Input: part model. Units: mm. Frame: model coordinates. Give positions to 0.01 mm unless a question says otherwise; leave off trailing zeros. Loops run counter-clockwise (first coordinate to the right, second up) from the corner with the lowest first, then second, coordinate; pieces in that order, holes last. Notation, with made-up numbers: M 35,53.5 L 92,53.5 A13 ccw 92,62.5 Z; hole C 1,40.25 d3. An arc over 180 degrees is marked long. Answer as a JSON object with one key per item and string values. Group by question number.
1) First-contact query: P1, Ø3, axis at x = 21.5, z = 0.5, coming from the -Y side; P2, Ø2, axis at y = -2, z = -0.5, coming from the +X side; P3, Ø3, axis at y = -1.5, z = 1.5, coming from the -X side; P4, Ø3, axis at x = 0, y = -2, coming from the +Z side. Flat tips, straight axial feed; report the tip coordinate or a pass-through.
2) Section query C-C on x = 24. Return loops of the section in (y, z), plus the area to 3 significant figures.
3) Section query A-A on z = 0. Return loops of the section in (x, y).
4) Draft query along Y for faces 1 (the cylindrical face through (9, 0, 2)), 2 (the flat face through (27.508, 1, 2)), 3 (the cylindrical face through (-9.03, -0.19, 0.03)). Return one class per face: +Y half, -Y half, draft (parallel to the pull), parting line (faces both ways), or undercut.
5) Section query B-B on y = 0. Return loops of the section in (x, z).
6) Ray query, L1, parallel to X at y = 0, z = -0.45; L2, parallel to X at y = 0, z = 1.2; L3, parallel to Y at x = 13, z = 0. Return the intervals inside material, ascending.
from build123d import *

# Parameters (mm, degrees)
SKETCH2_R          = 0.5
CUT_EXTRUDE1_DEPTH = 5
CHAMFER1_SIZE      = 0.5


with BuildPart() as part:
    # Sketch1 → Revolve1 (revolve)
    with BuildSketch(Plane.XY):
        with BuildLine():
            Line((-11.492242367, 0), (-11.492242367, -2))
            Line((-11.492242367, -2), (27.507757633, -2))
            Line((27.507757633, -2), (27.507757633, -3))
            ThreePointArc((27.507757633, -3), (29.629077976, -2.121320344), (30.507757633, 0))
            Line((30.507757633, 0), (-11.492242367, 0))
        make_face()
    revolve(axis=Axis((-20.421686747, 0, 0), (1, 0, 0)))

    # Sketch2 → Cut-Extrude1 (cut, symmetric)
    with BuildSketch(Plane.XY):
        with Locations((-9.492242367, 0)):
            Circle(SKETCH2_R)
    extrude(amount=CUT_EXTRUDE1_DEPTH, both=True, mode=Mode.SUBTRACT)

    # Chamfer1
    chamfer1_edges = [part.edges().sort_by_distance(p)[0] for p in [
        (-11.492242367, 2, 0),
    ]]
    chamfer(chamfer1_edges, length=CHAMFER1_SIZE)


solid = part.part
Output:
{
 "1": {"P1": "stops at y = -2", "P2": "stops at x = 30.31", "P3": "stops at x = -11.49", "P4": "stops at z = 1.94"},
 "2": {"outline": "C 0,0 d4", "area": "12.6 mm^2"},
 "3": {"outline": "M -11.49,-1.5 L -10.99,-2 L 27.51,-2 L 27.51,-3 A3 ccw 27.51,3 L 27.51,2 L -10.99,2 L -11.49,1.5 Z; hole C -9.49,0 d1"},
 "4": {"face 1": "parting line", "face 2": "draft", "face 3": "undercut"},
 "5": {"outline": "M -11.49,-1.5 L -10.99,-2 L -9.99,-2 L -9.99,2 L -10.99,2 L -11.49,1.5 Z; M -8.99,-2 L 27.51,-2 L 27.51,-3 A3 ccw 27.51,3 L 27.51,2 L -8.99,2 Z"},
 "6": {"L1": "x = -11.49 to -9.99, -8.99 to 30.47", "L2": "x = -11.49 to -9.99, -8.99 to 30.26", "L3": "y = -2 to 2"}
}
